Answer from the drawing. Dimensions are ordinates in mm from the lowest x, y and z of the part. A direction names the side the tool comes from. Coordinates: 2 decimals unless noted, no trailing zeros. Loops run counter-clockwise (first coordinate to the right, second up) from the corner with the lowest first, then second, coordinate; pieces in that order, holes last. Notation, with made-up numbers: M 21.5,85.5 L 54.5,85.5 A11 ccw 54.5,101.5 Z; hole C -19,28.5 d9. An arc over 180 degrees is marked long. Answer as CSV lines item,"result". Start each with the question number.
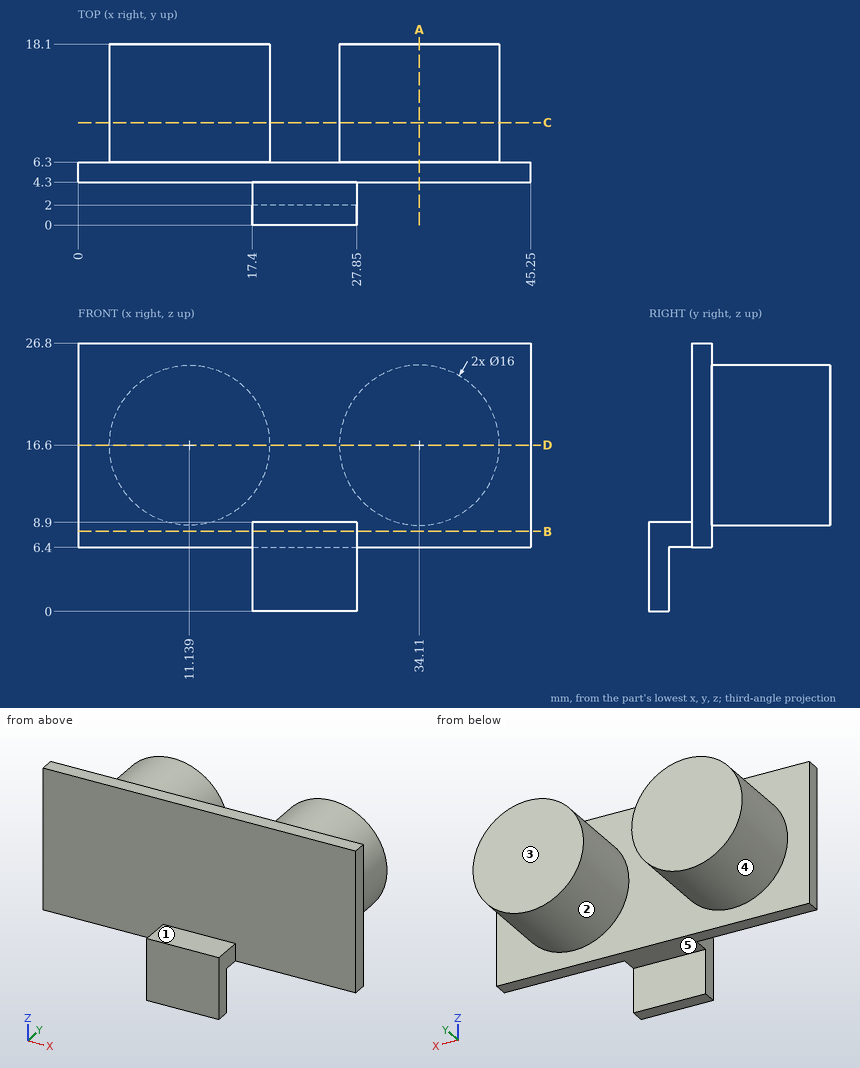
Item 1: Consider line 1 (Y direction, x = 23, z = 3.25); line 2 (X direction, y = 8.5, z = 19.25); line 3 (Y direction, x = 3, z = 14). Determine where each line is inside the solid, lowest interval first.
Item 2: For the marked faces 3, 4 and 5, determine the directions among +Z, -Z, +X, -X, +Y, -Y from which every point of the face is accessible in a straight line to the end or side of a thin tool.
Item 3: Section D-D on z = 16.6 is taken. Determine the outline of the cut face in (x, y), then the cut area to 3 significant figures.
Item 4: Each of these flat-tipped pins is pushed along its axis until it touches: P1, Ø1, axis at x = 37, z = 9.5, coming from the -Y side; P2, Ø2, axis at x = 16.5, y = 3.5, coming from the -Z side; P3, Ø1, axis at x = 30, y = 15.5, coming from the +Z side. Where does it stop, or does it pass through?
Item 5: For a pull along X with two mould halves and no side action, classify the marked faces 1 and 2 as pulls with the +X half, pulls with the -X half, needs draft (parallel to the pull), parting line crosses it, or undercut.
Item 6: Section C-C on y = 10.25 is taken. Determine the outline of the cut face in (x, z).
Item 7: Section A-A on x = 34.11 is taken. Determine the outline of the cut face in (y, z).
Item 8: Section B-B on z = 8 is taken. Determine the outline of the cut face in (x, y).
Results are:
1,line 1,"0 to 2"
1,line 2,"3.59 to 18.69, 26.56 to 41.66"
1,line 3,"4.3 to 6.3"
2,face 3,"+Z, -Z, +X, -X, +Y"
2,face 4,"+Y"
2,face 5,"-Z, +X, -X, +Y"
3,outline,"M 0,4.3 L 45.25,4.3 L 45.25,6.3 L 42.11,6.3 L 42.11,18.1 L 26.11,18.1 L 26.11,6.3 L 19.14,6.3 L 19.14,18.1 L 3.14,18.1 L 3.14,6.3 L 0,6.3 Z"
3,area,"468 mm²"
4,P1,"y = 4.3"
4,P2,"z = 6.4"
4,P3,"z = 23.74"
5,face 1,"needs draft"
5,face 2,"undercut"
6,outline,"C 11.14,16.6 d16; C 34.11,16.6 d16"
7,outline,"M 4.3,6.4 L 6.3,6.4 L 6.3,8.6 L 18.1,8.6 L 18.1,24.6 L 6.3,24.6 L 6.3,26.8 L 4.3,26.8 Z"
8,outline,"M 0,4.3 L 17.4,4.3 L 17.4,0 L 27.85,0 L 27.85,4.3 L 45.25,4.3 L 45.25,6.3 L 0,6.3 Z"
